Work out the finished part from the listing and answer in its coordinate system (mm). Face numbers are marked on the shaded views. A direction names the side the tool comes from. Coordinates: 2 decimals unless noted, no trailing zeros. Write each loop counter-clockwise with the first axis right and the second up, starting at its lowest first coordinate (ties: lowest second). Pieces come first, ordered by that corner, then holes. Notation, with made-up numbers: M -23.75,31 L 15.25,31 A24 ccw 15.25,51 Z; hole C -22.75,-13 d4. An arc over 180 degrees is marked long. Use CSV: the item, a comma, the result in double quotes.
from build123d import *

# Parameters (mm, degrees)
FLANGE_BASE1_DEPTH        = 5
FURO_ROSCADO_DE_M41_D     = 3.3
FURO_ROSCADO_DE_M42_D     = 3.3
QUEBRA_CANTO1_START       = -51.265241636
QUEBRA_CANTO1_OUTLINE_W   = 99.702056148
QUEBRA_CANTO1_OUTLINE_H   = 4
QUEBRA_CANTO1_DEPTH       = 1.414213562
QUEBRA_CANTO1_START_2     = 49.851028074
QUEBRA_CANTO1_2_OUTLINE_W = 99.702056148
QUEBRA_CANTO1_2_OUTLINE_H = 4
QUEBRA_CANTO1_2_DEPTH     = 1.414213562
QUEBRA_CANTO1_START_3     = -45.608387387
QUEBRA_CANTO1_3_OUTLINE_W = 2.148971926
QUEBRA_CANTO1_3_OUTLINE_H = 4
QUEBRA_CANTO1_3_DEPTH     = 91.216774774


# Read off the part's stored shape, not the designer's step: Quebra-Canto1
# Sheet-metal steps are written as plain solids
with BuildPart() as part:
    # Esboço1 → Flange-base1 (new, symmetric)
    with BuildSketch(Plane.XY):
        with BuildLine():
            Line((-67.5, 10), (-56.5, 10))
            ThreePointArc((-56.5, 10), (-53.671572875, 8.828427125), (-52.5, 6))
            Line((-52.5, 6), (-52.5, 2))
            ThreePointArc((-52.5, 2), (-51.914213562, 0.585786438), (-50.5, 0))
            Line((-50.5, 0), (50.5, 0))
            ThreePointArc((50.5, 0), (51.914213562, 0.585786438), (52.5, 2))
            Line((52.5, 2), (52.5, 6))
            ThreePointArc((52.5, 6), (53.671572875, 8.828427125), (56.5, 10))
            Line((56.5, 10), (67.5, 10))
            Line((67.5, 10), (67.5, 8))
            Line((67.5, 8), (56.5, 8))
            ThreePointArc((56.5, 8), (55.085786438, 7.414213562), (54.5, 6))
            Line((54.5, 6), (54.5, 2))
            ThreePointArc((54.5, 2), (53.328427125, -0.828427125), (50.5, -2))
            Line((50.5, -2), (-50.5, -2))
            ThreePointArc((-50.5, -2), (-53.328427125, -0.828427125), (-54.5, 2))
            Line((-54.5, 2), (-54.5, 6))
            ThreePointArc((-54.5, 6), (-55.085786438, 7.414213562), (-56.5, 8))
            Line((-56.5, 8), (-67.5, 8))
            Line((-67.5, 8), (-67.5, 10))
        make_face()
    extrude(amount=FLANGE_BASE1_DEPTH, both=True)

    # Furo roscado de M41 (through all)
    with Locations(Plane(origin=(0, -2, 0), x_dir=(-1, 0, 0), z_dir=(0, -1, 0))):
        with Locations((35, 0), (-35, 0)):
            Hole(FURO_ROSCADO_DE_M41_D / 2)

    # Furo roscado de M42 (through all)
    with Locations(Plane(origin=(0, 10, 0), x_dir=(1, 0, 0), z_dir=(0, 1, 0))):
        with Locations((-63.5, 0), (63.5, 0)):
            Hole(FURO_ROSCADO_DE_M42_D / 2)

    # Quebra-Canto1 outline → Quebra-Canto1 (cut)
    with BuildSketch(Plane(origin=(0, 0, 0), x_dir=(0.707106781186548, 0, 0.707106781186547), z_dir=(0.707106781186547, 0, -0.707106781186548)).offset(QUEBRA_CANTO1_START)):
        with Locations((0, -9)):
            Rectangle(QUEBRA_CANTO1_OUTLINE_W, QUEBRA_CANTO1_OUTLINE_H)
    extrude(amount=QUEBRA_CANTO1_DEPTH, mode=Mode.SUBTRACT)

    # Quebra-Canto1 2 outline → Quebra-Canto1 2 (cut)
    with BuildSketch(Plane(origin=(0, 0, 0), x_dir=(0.707106781186548, 0, 0.707106781186547), z_dir=(0.707106781186547, 0, -0.707106781186548)).offset(QUEBRA_CANTO1_START_2)):
        with Locations((0, -9)):
            Rectangle(QUEBRA_CANTO1_2_OUTLINE_W, QUEBRA_CANTO1_2_OUTLINE_H)
    extrude(amount=QUEBRA_CANTO1_2_DEPTH, mode=Mode.SUBTRACT)

    # Quebra-Canto1 3 outline → Quebra-Canto1 3 (cut)
    with BuildSketch(Plane(origin=(0, 0, 0), x_dir=(0.707106781186548, 0, 0.707106781186547), z_dir=(0.707106781186547, 0, -0.707106781186548)).offset(QUEBRA_CANTO1_START_3)):
        with Locations((-50.925514037, -9)):
            Rectangle(QUEBRA_CANTO1_3_OUTLINE_W, QUEBRA_CANTO1_3_OUTLINE_H)
        with Locations((50.925514037, -9)):
            Rectangle(QUEBRA_CANTO1_3_OUTLINE_W, QUEBRA_CANTO1_3_OUTLINE_H)
    extrude(amount=QUEBRA_CANTO1_3_DEPTH, mode=Mode.SUBTRACT)


solid = part.part
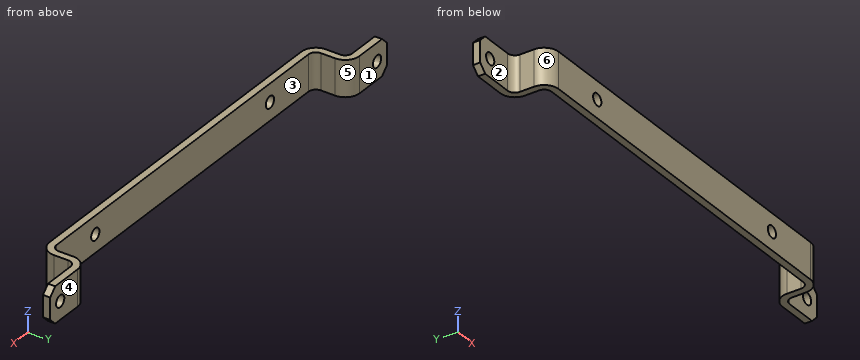
Item 1: A tool of negligible diameter and unlimited length cuts with its end or side. For the marked faces 1, 2 and 3, from which of +Z, -Z, +X, -X, +Y, -Y can it reach the whole face along a straight path? Write none if from no direction.
Answer:
face 1,"+Z, -Z, +X, -X, +Y"
face 2,"+Z, -Z, -X, -Y"
face 3,"+Z, -Z, +Y"
Item 2: Consider probe 1 along X at (y, z) = (2, 4.5); probe 2 along Z at (x, y) = (-63.5, 8.7); probe 3 along Y at (x, z) = (-44, -0.75). Determine where each line is inside the solid, lowest interval first.
Answer:
probe 1,"x = -54.5 to -52.5, 52.5 to 54.5"
probe 2,"z = -5 to -1.65, 1.65 to 5"
probe 3,"y = -2 to 0"
Item 3: The part is cut by section C-C (x = 42). Write down the section's boundary in (y, z).
Answer:
outline,"M -2,-5 L 0,-5 L 0,5 L -2,5 Z"
Item 4: The part is cut by section A-A (x = 63.5). Write down the section's boundary in (y, z), then the cut area to 3 significant figures.
Answer:
outline,"M 8,-5 L 10,-5 L 10,-1.65 L 8,-1.65 Z; M 8,1.65 L 10,1.65 L 10,5 L 8,5 Z"
area,"13.4 mm2"
Item 5: The part is cut by section B-B (y = 3.25). Write down the section's boundary in (x, z), then the cut area to 3 significant figures.
Answer:
outline,"M -54.5,-5 L -52.5,-5 L -52.5,5 L -54.5,5 Z; M 52.5,-5 L 54.5,-5 L 54.5,5 L 52.5,5 Z"
area,"40.0 mm2"
Item 6: Given pin 1 (5.5 mm diameter, centred on x = 63.5, z = 0, fed in from -Y); pin 2 (3 mm diameter, centred on y = 7.5, z = 2, fed in from -X); pin 3 (2 mm diameter, centred on y = 4.5, z = 1.5, fed in from -X); pin 4 (1.5 mm diameter, centred on x = -24.5, z = -0.5, fed in from +Y), each flat-ended and moving along its own axis, determine where each tip first touches the part or whether it passes through.
Answer:
pin 1,"stops at y = 8"
pin 2,"stops at x = -67.5"
pin 3,"stops at x = -54.5"
pin 4,"stops at y = 0"
Item 7: For a pull along X with two mould halves and no side action, classify the marked faces 4, 5 and 6 as released by +X, released by -X, zero draft, split by the parting line, or undercut.
Answer:
face 4,"zero draft"
face 5,"undercut"
face 6,"released by -X"
